Geometry check sheet. Reference: the model listing, model coordinates, mm. Give positions to 0.01 mm unless a question says otherwise; leave off trailing zeros. Order: outer loops, then holes, each group sorted by start corner. A loop starts at its lowest first (then second) coordinate and runs counter-clockwise, first axis right, second up.
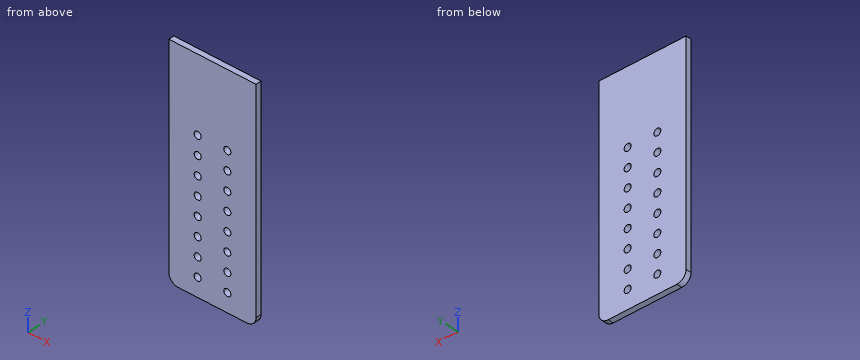
from build123d import *

# Parameters (mm, degrees)
CYLINDER002_R     = 1.9
CYLINDER002_DEPTH = 20
ARRAY003_Z_COUNT  = 8
ARRAY003_Z_PITCH  = 10
BOX003_W          = 47
BOX003_H          = 3
BOX003_DEPTH      = 120
FILLET003_R       = 5


with BuildPart() as laser_attachment_hole:
    # Cylinder002 → Cylinder002 (new body)
    with BuildSketch(Plane(origin=(8, 0, 0), x_dir=(1, 0, 0), z_dir=(0, -1, 0))):
        Circle(CYLINDER002_R)
    extrude(amount=CYLINDER002_DEPTH)


with BuildPart() as laser_hole_array:
    # Part__Mirroring003: instance of laser attachment hole
    add(laser_attachment_hole.part.mirror(Plane(origin=(0, 0, 0), x_dir=(0, -1, 0), z_dir=(1, 0, 0))))

    # Fusion002: union laser attachment hole
    add(laser_attachment_hole.part)

    # Array003 Z: laser hole array ×8


with BuildPart() as laser_hole_array_1:
    add(laser_hole_array.part)
    with Locations(*[(0, 0, i * ARRAY003_Z_PITCH) for i in range(1, ARRAY003_Z_COUNT)]):
        add(laser_hole_array.part)


with BuildPart() as laser_hole_array_2:
    # Array003 placement: moved
    add(laser_hole_array_1.part.moved(Location((0, 0, -5))))


with BuildPart() as holder_with_holes:
    # Box003 → Box003 (new body)
    with BuildSketch(Plane(origin=(-23.5, -11, -15), x_dir=(1, 0, 0), z_dir=(0, 0, 1))):
        with Locations((23.5, 1.5)):
            Rectangle(BOX003_W, BOX003_H)
    extrude(amount=BOX003_DEPTH)

    # Fillet003
    fillet003_edges = [holder_with_holes.edges().sort_by_distance(p)[0] for p in [
        (-23.5, -9.5, -15),
        (23.5, -9.5, -15),
    ]]
    fillet(fillet003_edges, radius=FILLET003_R)

    # Cut002: cut laser hole array
    add(laser_hole_array_2.part, mode=Mode.SUBTRACT)


solid = holder_with_holes.part
Item 1: Gauge pin test, flat end, axial feed: pin 1 (3.5 mm diameter, centred on x = 8, z = 65, fed in from +Y). Record the tip position at first contact, or that the pin passes through.
Reported:
pin 1: passes through
Item 2: Scan lines: L1, parallel to X at y = -10.35, z = 65; L2, parallel to Z at x = -19, y = -8.05; L3, parallel to Z at x = -20, y = -10.8. Record each from-to range of solid material in increasing order.
Reported:
L1: x = -23.5 to -9.9, -6.1 to 6.1, 9.9 to 23.5
L2: z = -14.97 to 105
L3: z = -14.77 to 105
Item 3: Sectioned sample at B-B (y = -9.25). Give the number of separate pieces and of enclosed holes in the cut face, and give its area (3 significant figures).
Reported:
separate pieces: 1
enclosed holes: 16
area: 5,450 mm2
Item 4: Sectioned sample at A-A (z = 65). Enter the section's corners in (x, y), and give its area (3 significant figures).
Reported:
outline: (-23.5, -11) - (-9.9, -11) - (-9.9, -8) - (-23.5, -8) - close; (-6.1, -11) - (6.1, -11) - (6.1, -8) - (-6.1, -8) - close; (9.9, -11) - (23.5, -11) - (23.5, -8) - (9.9, -8) - close
area: 118 mm2
